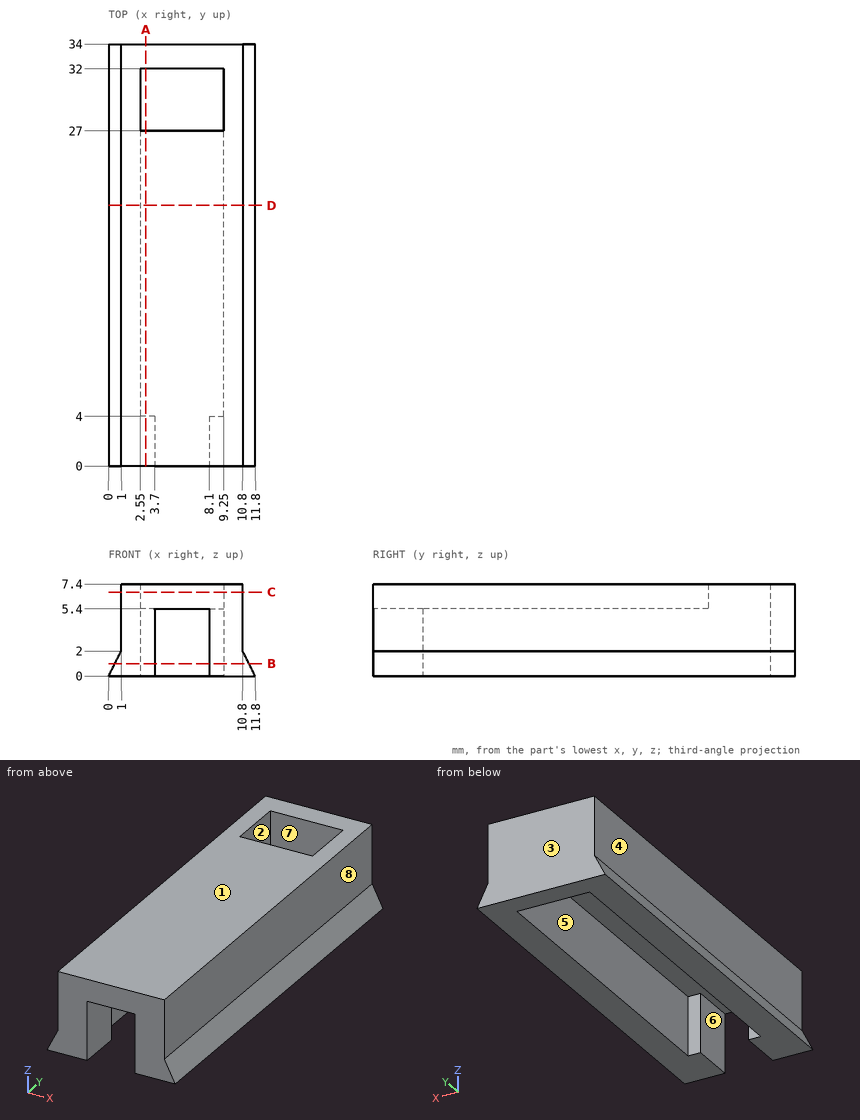
Can you work these out from the drawing? Everything is in mm from the part's minimum corner. A direction names the side the tool comes from. Give positions to 0.01 mm unless a question says otherwise; leave off trailing zeros. Order: outer loops, then holes, each group sorted by start corner. A loop starts at its lowest first (then second) coordinate and runs counter-clockwise, first axis right, second up. Notation, with made-up numbers: M 14.5,-19 L 39.5,-19 A6 ccw 39.5,-12 Z; hole C 84.25,35 d5. An arc over 180 degrees is marked long. Write item = value, one per line. Start each with the question number.
Q1. Suppose I cut it at C-C (z = 6.75). Write out the boundary of the cut face in (x, y), plus the area to 3 significant figures.
Q2. Suppose I cut it at B-B (z = 1). Write out the boundary of the cut face in (x, y), plus the area to 3 significant figures.
Q3. Will these pins go through, and if not, where does the flat tip stop? pin 1 Ø1.5 at (y, z) = (16.5, 2) entering from +X (3 decimals); pin 2 Ø2 at (y, z) = (2, 1.5) entering from +X; pin 3 Ø1.2 at (y, z) = (2.5, 4) entering from -X; pin 4 Ø2 at (x, z) = (6, 4.5) entering from -Y.
Q4. Suppose I cut it at A-A (x = 3). Write out the boundary of the cut face in (y, z).
Q5. We'd pull the mould along Y, two halves only. Please class the marked faces 1, 2 and 3: pulls with the +Y half, pulls with the -Y half, needs draft (parallel to the pull), parting line crosses it, or undercut.
Q6. Suppose I cut it at D-D (y = 21). Write out the boundary of the cut face in (x, z).
Q7. For the marked faces 4, 5, 6, 7 and 8, which set-ups out of +Z, -Z, +X, -X, +Y, -Y let a thin tool reach every point of the face, with its end or its side?
Q8. I need wall thicknesses on probe 1 along Y at (x, z) = (8.5, 3); probe 2 along X at (y, z) = (15, 3.75); probe 3 along Y at (x, z) = (6, 6.5). Which ranges of each line are inside material? Lowest first, please. Write a range as [from, to].
Check result:
q1.outline = M 1,0 L 10.8,0 L 10.8,34 L 1,34 Z; hole M 2.55,27 L 9.25,27 L 9.25,32 L 2.55,32 Z
q1.area = 300 mm2
q2.outline = M 0.5,0 L 3.7,0 L 3.7,4 L 2.55,4 L 2.55,32 L 9.25,32 L 9.25,4 L 8.1,4 L 8.1,0 L 11.3,0 L 11.3,34 L 0.5,34 Z
q2.area = 162 mm2
q3.pin_1 = 11.175
q3.pin_2 = 11.55
q3.pin_3 = 1
q3.pin_4 = 0
q4.outline = M 0,0 L 4,0 L 4,5.4 L 27,5.4 L 27,7.4 L 0,7.4 Z; M 32,0 L 34,0 L 34,7.4 L 32,7.4 Z
q5.face_1 = needs draft
q5.face_2 = undercut
q5.face_3 = pulls with the +Y half
q6.outline = M 0,0 L 2.55,0 L 2.55,5.4 L 9.25,5.4 L 9.25,0 L 11.8,0 L 10.8,2 L 10.8,7.4 L 1,7.4 L 1,2 Z
q7.face_4 = +Z, -X, +Y, -Y
q7.face_5 = -Z
q7.face_6 = -Z, -Y
q7.face_7 = +Z, -Z
q7.face_8 = +Z, +X, +Y, -Y
q8.probe_1 = [0, 4], [32, 34]
q8.probe_2 = [1, 2.55], [9.25, 10.8]
q8.probe_3 = [0, 27], [32, 34]
